The listing builds one solid part. Answer for the finished solid, in the listing's coordinates (mm). Face numbers are marked on the shaded views. Round coordinates to 2 decimals unless told otherwise and drop trailing zeros. Loops run counter-clockwise (first coordinate to the right, second up) from the corner with the lowest first, then second, coordinate; pieces in that order, holes last. Notation, with made-up numbers: (31.25, -13.5) - (37.25, -13.5) arc R14 cw to (37.25, 7.5) - close; hole circle Ø11 at (-24.75, 33.5). An arc over 180 degrees is marked (long way). One line per question, with ' | ' between items. Start each with the question number.
from build123d import *

# Parameters (mm, degrees)
F_0_1MM_FIT_FOR_POT_R   = 10.5
BOSS_EXTRUDE1_DEPTH     = 2.75
SKETCH4_R               = 10.5
SKETCH4_R_2             = 8.275
BOSS_EXTRUDE2_DEPTH     = 4.25
BOSS_EXTRUDE3_DEPTH     = 2
FILLET1_R               = 0.25
BOSS_EXTRUDE6_DEPTH     = 10
BOSS_EXTRUDE7_DEPTH     = 2.9
BOSS_EXTRUDE8_DEPTH     = 3
FILLET2_R               = 1.5
BOSS_EXTRUDE9_DEPTH     = 17.5
SKETCH11_W              = 12.5
SKETCH11_H              = 6
CUT_EXTRUDE1_DEPTH      = 76.428217957
CUT_EXTRUDE1_DEPTH_BACK = 76.428217957


with BuildPart() as part:
    # 0.1mm fit for pot → Boss-Extrude1 (new body)
    with BuildSketch(Plane(origin=(0, 0, 0), x_dir=(1, 0, 0), z_dir=(0, 1, 0))):
        with Locations(Location((0, 0, 0), (0, 0, 270))):
            Circle(F_0_1MM_FIT_FOR_POT_R)
    extrude(amount=BOSS_EXTRUDE1_DEPTH)

    # Sketch4 → Boss-Extrude2 (add)
    with BuildSketch(Plane(origin=(0, 2.75, 0), x_dir=(1, 0, 0), z_dir=(0, 1, 0))):
        with Locations(Location((0, 0, 0), (0, 0, 270))):
            Circle(SKETCH4_R)
        with Locations(Location((0, 0, 0), (0, 0, 270))):
            Circle(SKETCH4_R_2, mode=Mode.SUBTRACT)
    extrude(amount=BOSS_EXTRUDE2_DEPTH)

    # Sketch5 → Boss-Extrude3 (add)
    with BuildSketch(Plane(origin=(0, 2.75, 0), x_dir=(1, 0, 0), z_dir=(0, 1, 0))):
        with BuildLine():
            Line((-1, -8.214354813), (-1, -7.065799598))
            Line((-1, -7.065799598), (0.988059701, -7.065799598))
            Line((0.988059701, -7.065799598), (0.988059701, -8.215799598))
            ThreePointArc((0.988059701, -8.215799598), (-0.006013695, -8.274997815), (-1, -8.214354813))
        make_face()
    extrude(amount=BOSS_EXTRUDE3_DEPTH)

    # Fillet1
    fillet1_edges = [part.edges().sort_by_distance(p)[0] for p in [
        (0.988059701, 3.75, 7.065799598),
        (-1, 3.75, 7.065799598),
        (-0.005970149, 4.75, 7.065799598),
        (-1, 4.75, 7.640077205),
        (0.988059701, 4.75, 7.640799598),
    ]]
    fillet(fillet1_edges, radius=FILLET1_R)

    # Sketch7 → Boss-Extrude6 (add)
    with BuildSketch(Plane(origin=(0, 7, 0), x_dir=(1, 0, 0), z_dir=(0, 1, 0))):
        with BuildLine():
            Line((3.299602194, 9.968080325), (3.299602194, 8.373328213))
            ThreePointArc((3.299602194, 8.373328213), (-9, 0), (3.299602194, -8.373328213))
            Line((3.299602194, -8.373328213), (3.299602194, -9.968080325))
            ThreePointArc((3.299602194, -9.968080325), (-10.5, 0), (3.299602194, 9.968080325))
        make_face()
    extrude(amount=BOSS_EXTRUDE6_DEPTH)

    # Sketch8 → Boss-Extrude7 (add)
    with BuildSketch(Plane(origin=(0, 17, 0), x_dir=(1, 0, 0), z_dir=(0, 1, 0))):
        with BuildLine():
            Line((3.299602194, 12.315645552), (3.299602194, 9.968080325))
            ThreePointArc((3.299602194, 9.968080325), (-10.5, 0), (3.299602194, -9.968080325))
            Line((3.299602194, -9.968080325), (3.299602194, -12.315645552))
            ThreePointArc((3.299602194, -12.315645552), (-12.75, 0), (3.299602194, 12.315645552))
        make_face()
    extrude(amount=-BOSS_EXTRUDE7_DEPTH)

    # Sketch9 → Boss-Extrude8 (add)
    with BuildSketch(Plane.XZ):
        with BuildLine():
            Line((-9.3641604, 4.75), (-59.3641604, 4.75))
            Line((-59.3641604, 4.75), (-59.3641604, -4.75))
            Line((-59.3641604, -4.75), (-9.3641604, -4.75))
            ThreePointArc((-9.3641604, -4.75), (-10.5, 0), (-9.3641604, 4.75))
        make_face()
    extrude(amount=-BOSS_EXTRUDE8_DEPTH)

    # Fillet2
    fillet2_edges = [part.edges().sort_by_distance(p)[0] for p in [
        (-10.5, 3, 0),
        (-9.3641604, 1.5, 4.75),
        (-9.3641604, 1.5, -4.75),
    ]]
    fillet(fillet2_edges, radius=FILLET2_R)

    # Sketch10 → Boss-Extrude9 (add)
    with BuildSketch(Plane.ZY.offset(59.3641604)):
        with BuildLine():
            Line((-37.5, -19.5), (-35.5, -19.5))
            add(Edge.make_bspline(
                [(-4.75, 0), (-26.762186457, -1.948698647), (-35.5, -19.5)],
                knots=[0.548592822, 0.548592822, 0.548592822, 1, 1, 1], degree=2))
            Line((-4.75, 0), (4.75, 0))
            add(Edge.make_bspline(
                [(35.5, -19.5), (26.762186461, -1.948698647), (4.75, 0)],
                knots=[0, 0, 0, 0.451407178, 0.451407178, 0.451407178], degree=2))
            Line((35.5, -19.5), (37.5, -19.5))
            add(Edge.make_bspline(
                [(4.75, 3), (28.386779804, 0.912348176), (37.5, -19.5)],
                knots=[0.545557352, 0.545557352, 0.545557352, 1, 1, 1], degree=2))
            Line((4.75, 3), (-4.75, 3))
            add(Edge.make_bspline(
                [(-37.5, -19.5), (-28.386779803, 0.912348176), (-4.75, 3)],
                knots=[0, 0, 0, 0.454442648, 0.454442648, 0.454442648], degree=2))
        make_face()
    extrude(amount=-BOSS_EXTRUDE9_DEPTH)

    # Sketch11 → Cut-Extrude1 (cut, two sides)
    with BuildSketch(Plane(origin=(0, 0, -4.75), x_dir=(-1, 0, 0), z_dir=(0, 0, -1))) as cut_extrude1_sk:
        with Locations((50.6141604, -14.5)):
            Rectangle(SKETCH11_W, SKETCH11_H)
    extrude(amount=CUT_EXTRUDE1_DEPTH, mode=Mode.SUBTRACT)
    extrude(cut_extrude1_sk.sketch, amount=-CUT_EXTRUDE1_DEPTH_BACK, mode=Mode.SUBTRACT)


solid = part.part
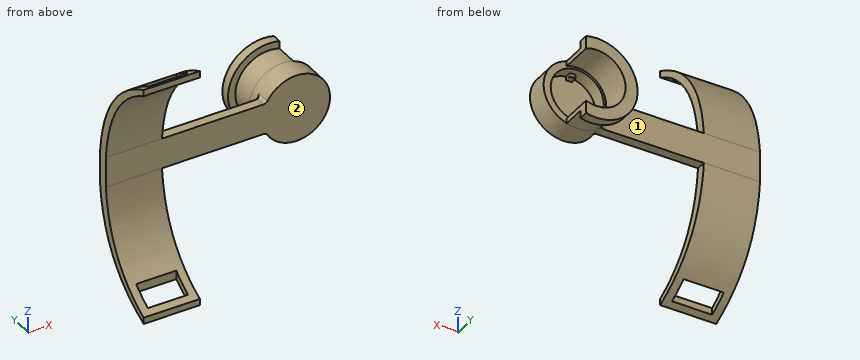
(1) Find section B-B on x = -50. Count the separate pieces of the cut face and the enclosed holes in it, plus the area to 3 significant figures.
(2) Find section A-A on z = 0. Write down the section's boundary in (x, y) (3 decimals).
(3) Consider L1, parallel to Z at x = 0, y = 5 (3 decimals); L2, parallel to Y at x = -1, z = 12; L3, parallel to X at y = -8.5, z = -28. Determine where each line is inside the solid, lowest interval first.
(4) Determine the mould class of the marked faces 1 and 2 for opening direction Z: pulls with the +Z half, pulls with the -Z half, needs draft (parallel to the pull), parting line crosses it, or undercut.
(5) Each of these flat-tipped pins is pushed along its axis until it touches: P1, Ø1.8, axis at y = -14.5, z = 33, coming from the +X side; P2, Ø5, axis at x = -41.5, z = 2.5, coming from the +Y side; P3, Ø1, axis at y = 3.5, z = 7.5, coming from the -X side; P4, Ø4, axis at y = -2.5, z = -3, coming from the +X side. Where does it stop, or does it pass through?
(6) Find section C-C on x = -40. Write down the section's boundary in (y, z), plus the area to 3 significant figures.
Answer below:
1) separate pieces: 3 | enclosed holes: 0 | area: 200 mm2
2) outline: (-59.364, 0) - (10.5, 0) - (10.5, 7) - (8.275, 7) - (8.275, 2.75) - (-8.275, 2.75) - (-8.275, 7) - (-9, 7) - (-9, 17) - (-12.75, 17) - (-12.75, 14.1) - (-10.5, 14.1) - (-10.5, 4.5) arc R1.5 cw to (-12, 3) - (-59.364, 3) - close
3) L1: -10.5 to -8.275, 8.275 to 10.5 | L2: 14.1 to 17 | L3: -59.36 to -41.86
4) face 1: needs draft | face 2: undercut
5) P1: x = -41.86 | P2: y = 3 | P3: x = -7.83 | P4: through
6) outline: (0, -4.75) - (3, -4.75) - (3, 4.75) - (0, 4.75) - close | area: 28.5 mm2
